Could you check a few things on this model? Use its own coordinates, in mm. A direction names the side the tool comes from. Give positions to 0.01 mm unless a question says otherwise; leave off trailing zeros. Loops run counter-clockwise (first coordinate to the right, second up) from the corner with the lowest first, then second, coordinate; pieces in that order, holes last. Notation, with made-up numbers: M 81.25,24.25 L 89.25,24.25 A7 cw 89.25,33.25 Z; hole C 7,-30.75 d1. An arc over 180 degrees is marked long. Answer in a Markdown table with one row per item. Add a question column.
1. Which directions (+Z, -Z, +X, -X, +Y, -Y) give clear straight access to the entire face, cutting with the end or side of a thin tool? Please do faces 5 (the cylindrical face through (19.55, 4.93, 22.43)), 6 (the cylindrical face through (-12.17, 5.72, -18.2)), 7 (the cylindrical face through (22.253, 1.479, 25.121)).
2. I need wall thicknesses on line 1 along Z through (x, y) = (5.5, 5.5); line 2 along X through (y, z) = (8.25, 10); line 3 along X through (y, z) = (4.25, 14). Which ranges of each line are inside material? Lowest first, please. Write a range as from..to.
3. If we section it at B-B on z = -15.5: List the corners of the cut face in (x, y) for me, then the cut area to 3 significant figures.
4. If we section it at A-A on x = -10: List the corners of the cut face in (y, z) for me, then the cut area to 3 significant figures.
5. I'm going to push flat-ended pins straight in: pin 1 Ø3 at (x, z) = (-24.5, 24) entering from +Y; pin 2 Ø0.8 at (x, y) = (24, 3.5) entering from +Z. Where does each tip first touch, or does it pass through?
6. If we section it at C-C on y = 5.5: Count the separate pieces of the cut face and the enclosed holes in it, then the cut area to 3 significant figures.
7. Thinking about a two-plate mould opening in X: for faces 1 (the cylindrical face through (-29.434, 5.07, 29.294)), 2 (the flat face through (0, 5, -32)), 3 (the cylindrical face through (29.434, 5.07, -29.294)), 4 (the cylindrical face through (2.89, 2.43, -18.2)), which applies, released by +X, released by -X, zero draft, split by the parting line, or undercut?
Autodesk Inventor part; units mm, degrees
ref_plane "Work Plane1" through (0, 5, 0) normal (0, 1, 0) x (1, 0, 0)
ref_plane "YZ Plane" through (0, 0, 0) normal (1, 0, 0) x (0, 1, 0)
ref_plane "XZ Plane" through (0, 0, 0) normal (0, 1, 0) x (-1, 0, 0)
sketch "Sketch1" plane through (0, 0, 0) normal (0, 1, 0) x (-1, 0, 0)
  line L0 (30, 30) -> (-30, 30)
  line L1 (-30, 30) -> (-30, -30)
  line L2 (-30, -30) -> (30, -30)
  line L3 (30, -30) -> (30, 30)
  line L4 (30, 30) -> (-30, -30) construction
  line L5 (-30, 30) -> (30, -30) construction
  point P0 (0, 0)
  dimension "d0" = 60
  dimension "d1" = 60
extrude "Extrusion1" add sketch "Sketch1" along normal blind 10
fillet "Fillet1" radius 7 4 edges at (30, 5, 30) (30, 5, -30) (-30, 5, 30) (-30, 5, -30)
sketch "Sketch2" plane through (0, 10, 0) normal (0, 1, 0) x (1, 0, 0)
  line L0 (-30, 30) -> (30, 30)
  line L1 (30, 30) -> (30, -30)
  line L2 (30, -30) -> (-30, -30)
  line L3 (-30, -30) -> (-30, 30)
  line L4 (-30, 30) -> (30, -30) construction
  line L5 (30, 30) -> (-30, -30) construction
  line L6 (25, -25) -> (25, 25)
  line L7 (25, 25) -> (-25, 25)
  line L8 (-25, 25) -> (-25, -25)
  line L9 (-25, -25) -> (25, -25)
  circle A0 centre (25, -25) radius 2.75
  circle A1 centre (-25, -25) radius 2.75
  circle A2 centre (25, 25) radius 2.75
  circle A3 centre (-25, 25) radius 2.75
  point P0 (0, 0)
  dimension "d5" = 5
  dimension "d6" = 5.5
  dimension "d7" = 5.5
  dimension "d8" = 5.5
  dimension "d9" = 5.5
extrude "Extrusion2" cut sketch "Sketch2" against normal blind 3 contours L9 A0 L6 | L6 A0 L9 | A2 L7 L6 | L6 L7 A2 | A1 L8 L9 | L9 L8 A1 | A3 L8 L7 | L7 L8 A3
sketch "Sketch3" plane through (0, 10, 0) normal (0, 1, 0) x (1, 0, 0)
  line L0 (-30, 30) -> (30, 30)
  line L1 (30, 30) -> (30, -30)
  line L2 (30, -30) -> (-30, -30)
  line L3 (-30, -30) -> (-30, 30)
  line L4 (-30, 30) -> (30, -30) construction
  line L5 (30, 30) -> (-30, -30) construction
  line L6 (20, -20) -> (20, 20.65)
  line L7 (-20, -20) -> (20, -20)
  line L8 (18, 18.65) -> (18, -18)
  line L9 (-20, 20.65) -> (20.65, 20.65)
  line L10 (18, 18.65) -> (18.65, 18.65)
  line L11 (-12.6, -18) -> (-12.6, 18.65)
  line L12 (-14.6, -20) -> (-14.6, 20.65)
  line L13 (18, 18.65) -> (-12.6, 18.65)
  line L14 (18, -18) -> (-12.6, -18)
  line L15 (-26, 20.65) -> (-20, 20.65)
  line L16 (-26, 20.65) -> (-26, -20)
  line L17 (-26, -20) -> (-20, -20)
  point P0 (0, 0)
  point P1 (-12.6, -20)
  dimension "d12" = 60
  dimension "d13" = 60
  dimension "d14" = 10
  dimension "d16" = 34.6
  dimension "d17" = 2
  dimension "d18" = 40.65
  dimension "d22" = 4
  dimension "d23" = 4
extrude "Extrusion3" cut sketch "Sketch3" against normal blind 2 contours L7 L12 L9 L6
sketch "Sketch4" plane through (0, 10, 0) normal (0, 1, 0) x (1, 0, 0)
  line L0 (-12.6, 18.65) -> (18, 18.65)
  line L1 (18, 18.65) -> (18, -18)
  line L2 (18, -18) -> (-12.6, -18)
  line L3 (-12.6, -18) -> (-12.6, 18.65)
  point P0 (0, 0)
extrude "Extrusion4" cut sketch "Sketch4" against normal blind 8
sketch "Sketch5" plane through (0, 10, 0) normal (0, 1, 0) x (1, 0, 0)
  line L0 (20, -20) -> (-14.6, -20)
  line L1 (-14.6, -20) -> (-14.6, 20.65)
  line L2 (-30, 23) -> (-30, -23)
  line L3 (-23, -30) -> (23, -30)
  line L4 (30, -23) -> (30, 23)
  line L5 (-26, 20.65) -> (-14.6, 20.65)
  line L6 (-26, -20) -> (-14.6, -20)
  line L7 (-26, 20.65) -> (-26, -20)
  line L8 (-14.6, -26) -> (-14.6, -20)
  line L9 (-14.6, -20) -> (-14.6, -26)
  line L10 (20, -26) -> (-14.6, -26)
  line L11 (20, -20) -> (20, -26)
  line L12 (26, -20) -> (20, -20)
  line L13 (26, 20.65) -> (20, 20.65)
  line L14 (30, -23) -> (30, 23)
  line L15 (26, 20.65) -> (26, -20)
  line L16 (23, 30) -> (-23, 30)
  line L17 (-14.6, 26) -> (-14.6, 20.65)
  line L18 (-14.6, 26) -> (20, 26)
  line L19 (20, 26) -> (20, 20.65)
  line L20 (-16.6, -20) -> (-16.6, 20.65)
  line L21 (20, -22) -> (-14.6, -22)
  line L22 (22, 20.65) -> (22, -20)
  line L23 (-14.6, 22.65) -> (18.1816, 22.65)
  line L24 (18.1816, 22.65) -> (20, 22.65)
  point P0 (0, 0)
  dimension "d28" = 4
  dimension "d29" = 4
  dimension "d30" = 4
  dimension "d31" = 4
  dimension "d32" = 4
  dimension "d33" = 4
  dimension "d36" = 4
  dimension "d37" = 4
  dimension "d38" = 2
  dimension "d39" = 2
extrude "Extrusion5" cut sketch "Sketch5" against normal through all contours L11 L10 L8 L21 | L22 L13 L15 L12 | L6 L7 L5 L20 | L17 L18 L19 L24 L23
fillet "Fillet2" radius 1.5 24 edges at (-16.6, 5, -20.65) (20, 5, -26) (26, 5, -20.65) (20, 5, 22) (-14.6, 5, -26) (-26, 5, -20.65) (22, 5, -20.65) (-14.6, 5, 22) (-26, 5, 20) (-14.6, 5, -22.65) (-14.6, 5, 26) (-16.6, 5, 20) (20, 5, 26) (26, 5, 20) (18, 2, -0.325) (2.7, 2, 18) (-12.6, 2, -0.325) (2.7, 2, -18.65) (-12.6, 5, -18.65) (18, 5, -18.65) (18, 5, 18) (-12.6, 5, 18) (22, 5, 20) (20, 5, -22.65)
sketch "Sketch6" plane through (-12.6, 3.5, 16.5) normal (1, 0, 0) x (0, 0, -1)
  point P0 (16.5, -3.5)
ref_plane "Work Plane1" through (0, 5, 0) normal (0, 1, 0) x (1, 0, 0)
mirror "Mirror1" about plane through (0, 5, 0) normal (0, 1, 0) of "Extrusion2"
sketch "Sketch7" plane through (0, 10, 0) normal (0, 1, 0) x (1, 0, 0)
  line L0 (-23, 30) -> (23, 30)
  line L1 (30, 23) -> (30, -23)
  line L2 (23, -30) -> (-23, -30)
  line L3 (-30, -23) -> (-30, 23)
  line L4 (-30, 30) -> (30, -30) construction
  line L5 (30, 30) -> (-30, -30) construction
  arc A0 (30, 23) -> (23, 30) centre (23, 23) ccw
  arc A1 (-23, 30) -> (-30, 23) centre (-23, 23) ccw
  arc A2 (-30, -23) -> (-23, -30) centre (-23, -23) ccw
  arc A3 (23, -30) -> (30, -23) centre (23, -23) ccw
  line L6 (32, -23) -> (32, 23)
  arc A4 (32, 23) -> (23, 32) centre (23, 23) ccw
  line L7 (23, 32) -> (-23, 32)
  arc A5 (-23, 32) -> (-32, 23) centre (-23, 23) ccw
  line L8 (-32, 23) -> (-32, -23)
  arc A6 (-32, -23) -> (-23, -32) centre (-23, -23) ccw
  line L9 (-23, -32) -> (23, -32)
  arc A7 (23, -32) -> (32, -23) centre (23, -23) ccw
  point P0 (0, 0)
  dimension "d45" = 60
  dimension "d46" = 60
  dimension "d47" = 7
  dimension "d48" = 2
extrude "Extrusion6" add sketch "Sketch7" against normal blind 10
properties part number "new IC holder"
Results:
| question | item | result |
|---|---|---|
| 1 | face 5 | +Y, -Y |
| 1 | face 6 | +Y |
| 1 | face 7 | -Y |
| 2 | line 1 | -32..-26, -22.65..-18.65, 18..22, 26..32 |
| 2 | line 2 | -32..-26, -16.6..-14.6, 20..22, 26..32 |
| 2 | line 3 | -32..-26, -16.6..-12.6, 18..22, 26..32 |
| 3 | outline | M -32,0 L -26,0 L -26,10 L -32,10 Z; M -16.6,0 L 22,0 L 22,10 L 20,10 L 20,8 L 18,8 L 18,3.5 A1.5 cw 16.5,2 L -11.1,2 A1.5 cw -12.6,3.5 L -12.6,8 L -14.6,8 L -14.6,10 L -16.6,10 Z; M 26,0 L 32,0 L 32,10 L 26,10 Z |
| 3 | area | 254 mm2 |
| 4 | outline | M 0,-32 L 10,-32 L 10,-26 L 0,-26 Z; M 0,-22.65 L 10,-22.65 L 10,-20.65 L 8,-20.65 L 8,-18.65 L 3.5,-18.65 A1.5 cw 2,-17.15 L 2,16.5 A1.5 cw 3.5,18 L 8,18 L 8,20 L 10,20 L 10,22 L 0,22 Z; M 0,26 L 10,26 L 10,32 L 0,32 Z |
| 4 | area | 266 mm2 |
| 5 | pin 1 | y = 7 |
| 5 | pin 2 | z = 31.98 |
| 6 | separate pieces | 1 |
| 6 | enclosed holes | 5 |
| 6 | area | 2,120 mm2 |
| 7 | face 1 | released by -X |
| 7 | face 2 | zero draft |
| 7 | face 3 | released by +X |
| 7 | face 4 | undercut |
